The figure shows three views and two pictorial views of one solid part (mm, origin at its lowest corner). Answer the questions. Round coordinates to 2 decimals unless told otherwise and drop trailing zeros. Write each loop counter-clockwise with the first axis right and the second up, starting at its lowest first coordinate (ties: lowest second). Pieces come first, ordered by that corner, then holes.
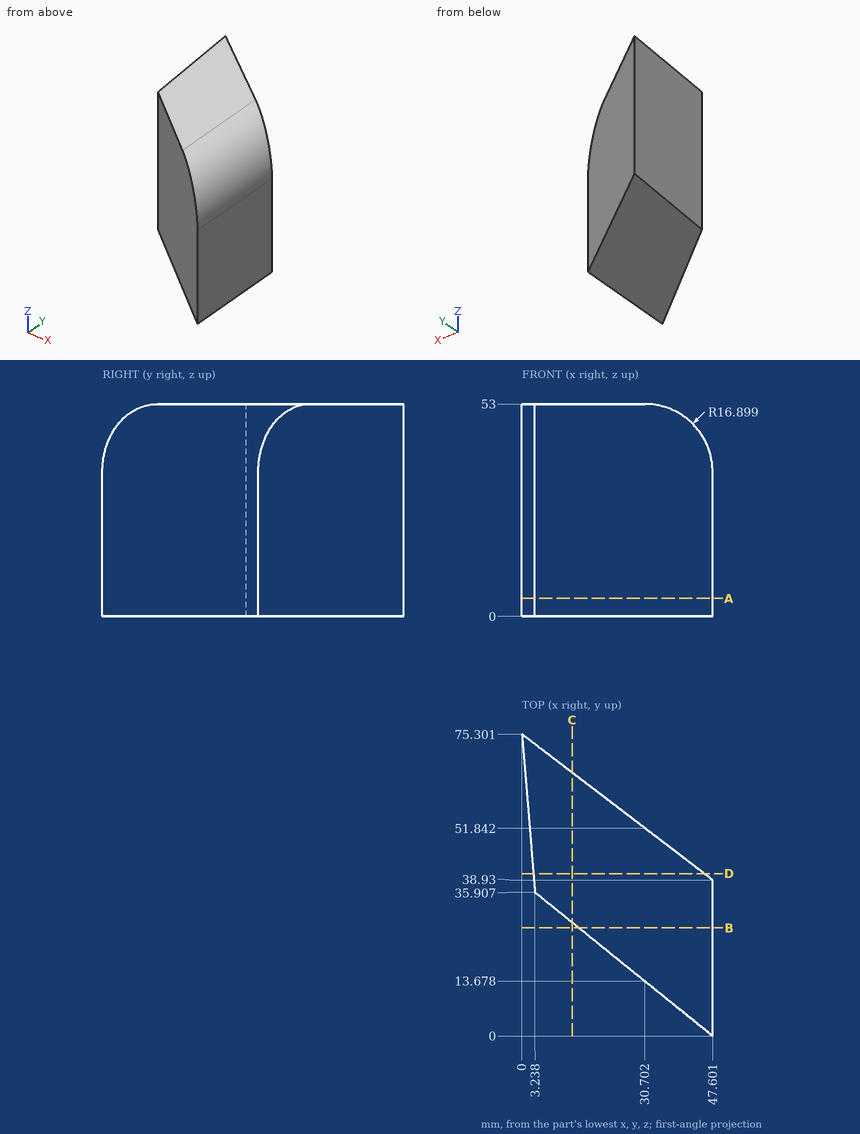
Q1. Section C-C (x = 12.5) is taken. Determine the outline of the cut face in (y, z), then the cut area to 3 significant figures.
Verdict:
outline: (28.41, 0) - (65.75, 0) - (65.75, 53) - (28.41, 53) - close
area: 1,980 mm2
Q2. Section A-A (z = 4.5) is taken. Determine the outline of the cut face in (x, y), then the cut area to 3 significant figures.
Verdict:
outline: (0, 75.3) - (3.24, 35.91) - (47.6, 0) - (47.6, 38.93) - close
area: 1,740 mm2
Q3. Flat-ended cylindrical pins translate along their axes: pin 1 Ø3 at (y, z) = (57.5, 47.5) entering from -X; pin 2 Ø5 at (y, z) = (54, 13) entering from +X; pin 3 Ø1.5 at (y, z) = (37, 37.5) entering from +X. Find the tip coordinate at first contact, or state that the pin passes through.
Verdict:
pin 1: stops at x = 1.34
pin 2: stops at x = 31.15
pin 3: stops at x = 47.59
Q4. Section B-B (y = 27) is taken. Determine the outline of the cut face in (x, z).
Verdict:
outline: (14.24, 0) - (47.6, 0) - (47.6, 36.1) arc R16.9 ccw to (30.7, 53) - (14.24, 53) - close
Q5. Straight lines are drawn through the part: probe 1 along Y at (x, z) = (35.5, 25) (1 decimal); probe 2 along Y at (x, z) = (42, 12) (1 decimal); probe 3 along X at (y, z) = (14, 22.5) (1 decimal). For each, find the intervals that lie inside material, in ascending order.
Verdict:
probe 1: y = 9.8 to 48.2
probe 2: y = 4.5 to 43.2
probe 3: x = 30.3 to 47.6
Q6. Section D-D (y = 40.5) is taken. Determine the outline of the cut face in (x, z).
Verdict:
outline: (2.86, 0) - (45.55, 0) - (45.55, 44.18) arc R16.9 ccw to (30.7, 53) - (2.86, 53) - close
